Input: part model. Units: mm. Frame: model coordinates. A direction names the side the tool comes from. Give positions to 0.01 mm unless a question says otherwise; leave off trailing zeros. Order: outer loops, then holes, each group sorted by start corner. A loop starts at its lowest first (then second) coordinate and runs counter-clockwise, first axis right, second up. Notation, with made-up numbers: (7, -20.5) - (32, -20.5) arc R20 cw to (32, 18.5) - close; hole circle Ø3 at (51.5, -12). An arc over 180 degrees is marked (long way). Use a Markdown table: item, result.
from build123d import *

# Parameters (mm, degrees)
F1_DEPTH = 25.4
F2_R     = 50.9875391609
F3_DEPTH = 38.1
F5_DEPTH = 38.1
F7_DEPTH = 25.4
F8_R     = 38.0488836494
F9_DEPTH = 63.5


with BuildPart() as f1:
    # F0 (on Top) → F1 (new body)
    with BuildSketch(Plane.XY):
        with BuildLine():
            Line((-60.883525759, 38.982976228), (-60.883525759, -37.2309312224))
            Line((-60.883525759, -37.2309312224), (17.0824285597, -37.2309312224))
            Line((17.0824285597, -37.2309312224), (17.0824285597, -36.4418395362))
            ThreePointArc((17.0824285597, -36.4418395362), (0.9326223834, 0.8760225028), (17.0824285597, 38.1938845418))
            Line((17.0824285597, 38.1938845418), (17.0824285597, 38.982976228))
            Line((17.0824285597, 38.982976228), (-60.883525759, 38.982976228))
        make_face()
        with BuildLine():
            Line((17.0824285597, 38.1938845418), (17.0824285597, -36.4418395362))
            ThreePointArc((17.0824285597, -36.4418395362), (72.4545517176, -46.1040347879), (103.313979079, 0.8760225028))
            ThreePointArc((103.313979079, 0.8760225028), (72.4545517176, 47.8560797934), (17.0824285597, 38.1938845418))
        make_face()
        with BuildLine():
            ThreePointArc((17.0824285597, 38.1938845418), (0.9326223834, 0.8760225028), (17.0824285597, -36.4418395362))
            Line((17.0824285597, -36.4418395362), (17.0824285597, 38.1938845418))
        make_face()
    extrude(amount=F1_DEPTH)

    # F2 (on face) → F3 (join)
    with BuildSketch(Plane.XY.offset(25.4)):
        with Locations((52.1233007312, 0.8760225028)):
            Circle(F2_R)
    extrude(amount=F3_DEPTH)

    # F4 (on face) → F5 (join)
    with BuildSketch(Plane.XY.offset(25.4)):
        with BuildLine():
            Line((1.311869915, 5.1101278514), (-60.883525759, 5.1101278514))
            Line((-60.883525759, 5.1101278514), (-60.883525759, -5.1101278514))
            Line((-60.883525759, -5.1101278514), (0, -5.1101278514))
            Line((0, -5.1101278514), (1.311869915, -5.1101278514))
            Line((1.311869915, -5.1101278514), (1.311869915, -3.3580828458))
            ThreePointArc((1.311869915, -3.3580828458), (1.1357615703, 0.8760225028), (1.311869915, 5.1101278514))
        make_face()
    extrude(amount=F5_DEPTH)

    # F6 (on face) → F7 (cut)
    with BuildSketch(Plane.XZ.offset(5.1101278514)):
        Polygon((-60.883525759, 63.5), (-60.883525759, 25.4), (1.311869915, 63.5), align=None)
    extrude(amount=-F7_DEPTH, mode=Mode.SUBTRACT)

    # F8 (on face) → F9 (cut)
    with BuildSketch(Plane.XY.offset(63.5)):
        with Locations((52.1233007312, 0.8760225028)):
            Circle(F8_R)
    extrude(amount=-F9_DEPTH, mode=Mode.SUBTRACT)


solid = f1.part
1. Material intervals for line 1 along Y through (x, z) = (-9.5, 7); line 2 along Y through (x, z) = (33.5, 51); line 3 along Z through (x, y) = (-21.5, 17.5), sorted ascending.
Response:
| item | result |
|---|---|
| line 1 | y = -37.23 to 38.98 |
| line 2 | y = -46.59 to -32.3, 34.06 to 48.34 |
| line 3 | z = 0 to 25.4 |
2. Section query B-B (x = 83). Return loops of the section in (y, z).
Response:
| item | result |
|---|---|
| outline | (-39.95, 0) - (-21.36, 0) - (-21.36, 63.5) - (-39.7, 63.5) - (-39.7, 25.4) - (-39.95, 25.4) - close; (23.11, 0) - (41.71, 0) - (41.71, 25.4) - (41.45, 25.4) - (41.45, 63.5) - (23.11, 63.5) - close |
3. Pin query (flat end, axial travel): pin 1 (0.6 mm diameter, centred on y = 38.5, z = 11, fed in from +X); pin 2 (3 mm diameter, centred on y = 9.5, z = 48.5, fed in from +X); pin 3 (11.5 mm diameter, centred on x = -21, z = 40, fed in from +Y). Return the tip coordinate at first contact, or that it passes through.
Response:
| item | result |
|---|---|
| pin 1 | stops at x = 87.16 |
| pin 2 | stops at x = 102.61 |
| pin 3 | stops at y = 5.11 |
4. Set-up query: faces 1 (the face through (14, -6, 63.5)), 2 (the face through (-22, -37.231, 13)), 3 (the face through (-22, 5.11, 40)), 4 (the face through (-21, 38.983, 13)), 5 (the face through (-16, -5.11, 36)). Return all of +Z, -Z, +X, -X, +Y, -Y with unobstructed straight access to the full face (end or side cutting, diameter ignored); none if empty.
Response:
| item | result |
|---|---|
| face 1 | +Z, +X, -X, +Y, -Y |
| face 2 | +Z, -Z, -X, -Y |
| face 3 | +Z, -X, +Y |
| face 4 | +Z, -Z, -X, +Y |
| face 5 | +Z, -X, -Y |
5. Section query A-A (z = 13.5). Return loops of the section in (x, y), then the cut area to 3 significant figures.
Response:
| item | result |
|---|---|
| outline | (-60.88, -37.23) - (17.08, -37.23) - (17.08, -36.44) arc R51.19 ccw (long way) to (17.08, 38.19) - (17.08, 38.98) - (-60.88, 38.98) - close; hole circle Ø76.1 at (52.12, 0.88) |
| area | 8,790 mm^2 |
6. Section query D-D (x = -11.5). Return loops of the section in (y, z).
Response:
| item | result |
|---|---|
| outline | (-37.23, 0) - (38.98, 0) - (38.98, 25.4) - (5.11, 25.4) - (5.11, 55.65) - (-5.11, 55.65) - (-5.11, 25.4) - (-37.23, 25.4) - close |
7. Section query C-C (y = -28). Return loops of the section in (x, z), then the cut area to 3 significant figures.
Response:
| item | result |
|---|---|
| outline | (-60.88, 0) - (27.35, 0) - (27.35, 63.5) - (10.1, 63.5) - (10.1, 25.4) - (-60.88, 25.4) - close; (76.9, 0) - (94.39, 0) - (94.39, 25.4) - (94.15, 25.4) - (94.15, 63.5) - (76.9, 63.5) - close |
| area | 4,000 mm^2 |
